Autodesk Fusion 360 part; units mm, degrees
sketch "Schizzo1" plane through (0, 0, 0) normal (0, 0, 1) x (1, 0, 0)
  line L0 (-42.5691, 59.0067) -> (24.1309, 59.0067) construction
  line L1 (24.1309, 59.0067) -> (24.1309, 5.3067) construction
  line L2 (24.1309, 5.3067) -> (-42.5691, 5.3067) construction
  line L3 (-42.5691, 5.3067) -> (-42.5691, 59.0067) construction
  line L4 (24.0309, 58.9067) -> (24.0309, 5.4067)
  line L5 (24.0309, 5.4067) -> (-42.4691, 5.4067)
  line L6 (-42.4691, 5.4067) -> (-42.4691, 58.9067)
  line L7 (-42.4691, 58.9067) -> (24.0309, 58.9067)
  line L8 (22.1309, 7.3067) -> (-40.5691, 7.3067)
  line L9 (-40.5691, 7.3067) -> (-40.5691, 57.0067)
  line L10 (-40.5691, 57.0067) -> (22.1309, 57.0067)
  line L11 (22.1309, 57.0067) -> (22.1309, 7.3067)
  line L12 (-40.5691, 57.0067) -> (-12.5691, 57.0067)
  line L13 (-12.5691, 57.0067) -> (-12.5691, 47.0067)
  line L14 (-12.5691, 47.0067) -> (-40.5691, 47.0067)
  line L15 (-40.5691, 47.0067) -> (-40.5691, 57.0067)
  line L16 (-42.5691, 32.1567) -> (24.1309, 32.1567) construction
  line L17 (-9.2191, 59.0067) -> (-9.2191, 5.3067) construction
  line L18 (-40.5691, 37.1567) -> (22.1309, 37.1567)
  line L19 (-40.5691, 27.1567) -> (22.1309, 27.1567)
  dimension "d1" = 66.7
  dimension "d2" = 53.7
  dimension "d3" = 0.1
  dimension "d8" = 2
  dimension "d9" = 28
  dimension "d10" = 10
  dimension "d11" = 10
extrude "Estrusione1" add sketch "Schizzo1" along normal blind 4 contours L8 L9 L11 L19 | L9 L11 L18 L19 | L9 L10 L11 L13 L14 L18
extrude "Estrusione4" add sketch "Schizzo1" along normal blind 2
fillet "Raccordo1" radius 2 4 edges at (-42.4691, 5.4067, 1) (24.0309, 5.4067, 1) (24.0309, 58.9067, 1) (-42.4691, 58.9067, 1)
extrude "Estrusione2" cut sketch "Schizzo1" against normal blind 3 from surface at 4 contours L8 L9 L11 L19 | L9 L10 L11 L13 L14 L18
ref_plane "Piano di lavoro1" through (-9.2191, 32.1567, 0) normal (1, 0, 0) x (0, -1, 0)
sketch "Schizzo2" plane through (-9.2191, 0, 0) normal (1, 0, 0) x (0, 1, 0)
  line L0 (5.4067, 4) -> (58.9067, 4) construction
  line L1 (58.9067, 4) -> (58.9067, 0) construction
  line L2 (58.9067, 0) -> (5.4067, 0) construction
  line L3 (5.4067, 0) -> (5.4067, 4) construction
  line L4 (58.9067, 2) -> (58.9067, 0) construction
  line L5 (7.4067, 0) -> (56.9067, 0) construction
  line L6 (5.4067, 0) -> (5.4067, 2) construction
  line L7 (37.1567, 4) -> (27.1567, 4) construction
  line L8 (32.1567, 4) -> (32.1567, 0) construction
  line L9 (27.1567, 4) -> (27.1567, 0) construction
  line L10 (27.1567, 2) -> (27.1567, 4) construction
  line L11 (5.4067, 1) -> (58.9067, 1) construction
  line L12 (7.3067, 1) -> (27.1567, 1) construction
  line L13 (37.1567, 4) -> (37.1567, 0) construction
  line L14 (27.1567, 4) -> (28.8887, 1)
  line L15 (27.1567, 4) -> (30.6208, 4) construction
  line L16 (28.8887, 1) -> (27.1567, 1)
  line L17 (27.1567, 1) -> (27.1567, 4)
  line L18 (37.1567, 4) -> (35.4246, 1)
  line L19 (37.1567, 1) -> (37.1567, 4)
  line L20 (35.4246, 1) -> (37.1567, 1)
  dimension "d24" = 60
extrude "Estrusione3" cut sketch "Schizzo2" along normal mid plane 60
Geometry: final body of the model. Coordinates: model frame, mm. A direction names the side the tool comes from. Round coordinates to 2 decimals unless told otherwise and drop trailing zeros. Loops run counter-clockwise (first coordinate to the right, second up) from the corner with the lowest first, then second, coordinate; pieces in that order, holes last.
Q1. Section A-A on x = -15. Return loops of the section in (y, z), plus the area to 3 significant figures.
Q2. Access query for faces 4 (the flat face through (20.781, 37, 2)), 5 (the cylindrical face through (23.461, 58.305, 1.014)), 6 (the flat face through (21, 37.157, 3)). Directions: +Z, -Z, +X, -X, +Y, -Y. A direction counts if a zero-diameter tool reaches every point of the face in a straight line with its end or side. Return the directions, or none.
Q3. Pull-direction query (X, two-part tool) for faces 1 (the cylindrical face through (-41.9, 6.01, 1.01)), 2 (the flat face through (-10, 18, 1)), 3 (the flat face through (-9, 5.407, 1)); classes: released by +X, released by -X, zero draft, split by the parting line, or undercut.
Q4. Section D-D on y = 50. Return loops of the section in (x, z).
Q5. Material intervals for L1, parallel to X at y = 56.5, z = 0.65; L2, parallel to X at y = 12, z = 1.3; L3, parallel to Z at x = -25.5, y = 44.5, sorted ascending.
Q6. Pin query (flat end, axial travel): P1, Ø1.1, axis at x = -40, z = 3, coming from the +Y side; P2, Ø0.7, axis at x = 21.5, z = 3, coming from the -Y side; P3, Ø1, axis at y = 34, z = 3, coming from the +X side; P4, Ø2, axis at x = -22, y = 45.5, coming from the -Z side. Return the tip coordinate at first contact, or that it passes through.
Q7. Section C-C on x = 6. Return loops of the section in (y, z), plus the area to 3 significant figures.
Q8. Section B-B on y = 31. Return loops of the section in (x, z), plus the area to 3 significant figures.
Evaluation:
1. outline: (5.41, 0) - (47.01, 0) - (47.01, 1) - (35.42, 1) - (37.16, 4) - (27.16, 4) - (28.89, 1) - (7.31, 1) - (7.31, 2) - (5.41, 2) - close; (57.01, 0) - (58.91, 0) - (58.91, 2) - (57.01, 2) - close
1. area: 72.1 mm2
2. face 4: none
2. face 5: +Z, -Z, +X, +Y
2. face 6: +Z
3. face 1: released by -X
3. face 2: undercut
3. face 3: zero draft
4. outline: (-42.47, 0) - (-40.57, 0) - (-40.57, 2) - (-42.47, 2) - close; (-12.57, 0) - (24.03, 0) - (24.03, 2) - (22.13, 2) - (22.13, 1) - (-12.57, 1) - close
5. L1: x = -42.47 to -40.57, -12.57 to 24.03
5. L2: x = -42.47 to -40.57, 22.13 to 24.03
5. L3: z = 0 to 1
6. P1: stops at y = 37.16
6. P2: stops at y = 27.16
6. P3: stops at x = 22.13
6. P4: stops at z = 0
7. outline: (5.41, 0) - (58.91, 0) - (58.91, 2) - (57.01, 2) - (57.01, 1) - (35.42, 1) - (37.16, 4) - (27.16, 4) - (28.89, 1) - (7.31, 1) - (7.31, 2) - (5.41, 2) - close
7. area: 82.1 mm2
8. outline: (-42.47, 0) - (24.03, 0) - (24.03, 2) - (22.13, 2) - (22.13, 4) - (-40.57, 4) - (-40.57, 2) - (-42.47, 2) - close
8. area: 258 mm2
